Autodesk Inventor part; units mm, degrees
ref_plane "YZ Plane" through (0, 0, 0) normal (1, 0, 0) x (0, 1, 0)
ref_plane "XZ Plane" through (0, 0, 0) normal (0, 1, 0) x (-1, 0, 0)
ref_plane "XY Plane" through (0, 0, 0) normal (0, 0, 1) x (1, 0, 0)
sketch "Sketch1" plane through (0, 0, 0) normal (0, 1, 0) x (-1, 0, 0)
  line L0 (24.925, 14.925) -> (-24.925, 14.925)
  line L1 (-24.925, 14.925) -> (-24.925, -14.925)
  line L2 (-24.925, -14.925) -> (24.925, -14.925)
  line L3 (24.925, 14.925) -> (-24.925, -14.925) construction
  line L4 (-24.925, 14.925) -> (24.925, -14.925) construction
  line L5 (24.925, -14.925) -> (24.925, 14.925)
  line L6 (24.925, 5) -> (24.925, 14.925)
  point P0 (0, 0)
  dimension "d0" = 49.85
  dimension "d1" = 29.85
extrude "Extrusion1" add sketch "Sketch1" along normal blind 1.4
sketch "Sketch2" plane through (0, 0, 0) normal (0, -1, 0) x (1, 0, 0)
  point P0 (0, 0)
sketch "Sketch3" plane through (-24.925, 0, -14.925) normal (-1, 0, 0) x (0, 0, 1)
  point P0 (14.925, 0)
ref_plane "Work Plane1" through (0, 0, 0) normal (0, 1, 0) x (-1, 0, 0)
sketch "Sketch5" plane through (0, 0, 0) normal (0, 1, 0) x (-1, 0, 0)
  line L0 (-24.925, 14.925) -> (24.925, 14.925)
  line L1 (24.925, -14.925) -> (-24.925, -14.925)
  line L2 (24.925, 14.925) -> (24.925, -14.925)
  line L3 (-19.3821, 7.7039) -> (19.3821, 7.7039) construction
  line L4 (19.3821, 7.7039) -> (19.3821, -7.7039) construction
  line L5 (19.3821, -7.7039) -> (-19.3821, -7.7039) construction
  line L6 (-19.3821, -7.7039) -> (-19.3821, 7.7039) construction
  line L7 (-24.925, -14.925) -> (-24.925, 14.925)
  line L8 (-12.5833, 1.3105) -> (-16.2231, 1.3105)
  line L9 (-16.2231, 1.3105) -> (-16.2231, 3.7476)
  spline S0 degree 2 poles (-16.2231, 3.7476) (-16.2231, 4.8026) (-16.4552, 5.3301) (-16.8561, 5.3301) knots 0 0 0 1 2 2 2
  spline S1 degree 2 poles (-16.8561, 5.3301) (-17.3097, 5.3301) (-17.5524, 4.6866) (-17.5524, 3.6316) knots 0 0 0 1 2 2 2
  line L10 (-17.5524, 3.6316) -> (-17.5524, -2.8673)
  spline S2 degree 2 poles (-17.5524, -2.8673) (-17.5524, -3.8907) (-17.3097, -4.5131) (-16.8877, -4.5131) knots 0 0 0 1 2 2 2
  spline S3 degree 2 poles (-16.8877, -4.5131) (-16.4763, -4.5131) (-16.2231, -3.8907) (-16.2231, -2.7407) knots 0 0 0 1 2 2 2
  line L11 (-16.2231, -2.7407) -> (-16.2231, -0.9788)
  line L12 (-16.2231, -0.9788) -> (-12.5833, -0.9788)
  line L13 (-12.5833, -0.9788) -> (-12.5833, -1.5274)
  spline S4 degree 2 poles (-12.5833, -1.5274) (-12.5833, -3.7008) (-13.1952, -5.5154) (-15.3052, -6.8869) (-16.835, -6.8869) knots 0 0 0 1 2 3 3 3
  spline S5 degree 2 poles (-16.835, -6.8869) (-18.4386, -6.8869) (-20.517, -5.7264) (-21.1922, -3.6797) (-21.1922, -1.6224) knots 0 0 0 1 2 3 3 3
  line L14 (-21.1922, -1.6224) -> (-21.1922, 2.4711)
  spline S6 degree 2 poles (-21.1922, 2.4711) (-21.1922, 3.9797) (-20.9812, 5.4989) (-19.9578, 6.9021) (-18.1326, 7.7039) (-16.9405, 7.7039) knots 0 0 0 1 2 3 4 4 4
  spline S7 degree 2 poles (-16.9405, 7.7039) (-15.3369, 7.7039) (-13.2374, 6.459) (-12.5833, 4.6022) (-12.5833, 2.6399) knots 0 0 0 1 2 3 3 3
  line L15 (-12.5833, 2.6399) -> (-12.5833, 1.3105)
  line L16 (-11.2751, 7.4085) -> (-8.7008, 7.4085)
  spline S8 degree 2 poles (-8.7008, 7.4085) (-6.1266, 7.4085) (-4.3014, 7.0076) (-3.1515, 5.3723) (-3.1515, 3.5894) knots 0 0 0 1 2 3 3 3
  spline S9 degree 2 poles (-3.1515, 3.5894) (-3.1515, 1.9541) (-3.9638, 0.8252) (-5.156, 0.7092) knots 0 0 0 1 2 2 2
  spline S10 degree 2 poles (-5.156, 0.7092) (-4.0799, 0.4454) (-3.3308, -0.4513) (-3.1515, -1.2004) (-3.1515, -2.899) knots 0 0 0 1 2 3 3 3
  line L17 (-3.1515, -2.899) -> (-3.1515, -6.5915)
  line L18 (-3.1515, -6.5915) -> (-6.5381, -6.5915)
  line L19 (-6.5381, -6.5915) -> (-6.5381, -1.9389)
  spline S11 degree 2 poles (-6.5381, -1.9389) (-6.5381, -0.8206) (-6.8862, -0.2825) (-7.6353, -0.2825) knots 0 0 0 1 2 2 2
  line L20 (-7.6353, -0.2825) -> (-7.6353, -6.5915)
  line L21 (-7.6353, -6.5915) -> (-11.2751, -6.5915)
  line L22 (-11.2751, -6.5915) -> (-11.2751, 7.4085)
  line L23 (-7.6353, 5.0136) -> (-7.6353, 1.9013)
  spline S12 degree 2 poles (-7.6353, 1.9013) (-7.0234, 1.9013) (-6.5381, 2.239) (-6.5381, 3.1674) knots 0 0 0 1 2 2 2
  line L24 (-6.5381, 3.1674) -> (-6.5381, 3.9375)
  spline S13 degree 2 poles (-6.5381, 3.9375) (-6.5381, 4.6022) (-7.0128, 5.0136) (-7.6353, 5.0136) knots 0 0 0 1 2 2 2
  line L25 (4.5501, 7.4085) -> (6.639, -6.5915)
  line L26 (6.639, -6.5915) -> (2.9043, -6.5915)
  line L27 (2.9043, -6.5915) -> (2.7144, -4.07)
  line L28 (2.7144, -4.07) -> (1.4167, -4.07)
  line L29 (1.4167, -4.07) -> (1.2057, -6.5915)
  line L30 (1.2057, -6.5915) -> (-2.5712, -6.5915)
  line L31 (-2.5712, -6.5915) -> (-0.725, 7.4085)
  line L32 (-0.725, 7.4085) -> (4.5501, 7.4085)
  spline S14 degree 2 poles (2.6194, -1.5907) (2.3557, 0.783) (2.0708, 4.2857) knots 0 0 0 1 1 1
  spline S15 degree 2 poles (2.0708, 4.2857) (1.5222, 0.2661) (1.3745, -1.5907) knots 0 0 0 1 1 1
  line L33 (1.3745, -1.5907) -> (2.6194, -1.5907)
  line L34 (7.2615, 7.4085) -> (10.9329, 7.4085)
  spline S16 degree 2 poles (10.9329, 7.4085) (12.4205, 7.4085) (14.0241, 6.9443) (14.8259, 6.0581) (15.1108, 4.8026) (15.1108, 3.4944) knots 0 0 0 1 2 3 4 4 4
  line L35 (15.1108, 3.4944) -> (15.1108, 2.2706)
  spline S17 degree 2 poles (15.1108, 2.2706) (15.1108, 0.9307) (14.5516, -0.3036) (13.0746, -0.9577) (11.8824, -0.9577) knots 0 0 0 1 2 3 3 3
  line L36 (11.8824, -0.9577) -> (10.9013, -0.9577)
  line L37 (10.9013, -0.9577) -> (10.9013, -6.5915)
  line L38 (10.9013, -6.5915) -> (7.2615, -6.5915)
  line L39 (7.2615, -6.5915) -> (7.2615, 7.4085)
  line L40 (10.9013, 5.0136) -> (10.9013, 1.4477)
  spline S18 degree 2 poles (10.9013, 1.4477) (11.0595, 1.4371) (11.165, 1.4371) knots 0 0 0 1 1 1
  spline S19 degree 2 poles (11.165, 1.4371) (11.6714, 1.4371) (12.0618, 1.933) (12.0618, 2.7137) knots 0 0 0 1 2 2 2
  line L41 (12.0618, 2.7137) -> (12.0618, 3.8637)
  spline S20 degree 2 poles (12.0618, 3.8637) (12.0618, 4.5811) (11.6081, 5.0136) (10.9013, 5.0136) knots 0 0 0 1 2 2 2
  line L42 (19.6704, 7.4085) -> (19.4094, -2.7341)
  line L43 (19.4094, -2.7341) -> (17.8551, -2.7341)
  line L44 (17.8551, -2.7341) -> (17.5715, 7.4085)
  line L45 (17.5715, 7.4085) -> (19.6704, 7.4085)
  line L46 (19.5796, -6.5915) -> (17.6623, -6.5915)
  line L47 (17.6623, -6.5915) -> (17.6623, -4.6061)
  line L48 (17.6623, -4.6061) -> (19.5796, -4.6061)
  line L49 (19.5796, -4.6061) -> (19.5796, -6.5915)
  point P0 (0, 0)
  dimension "d13" = 29.85
  dimension "d14" = 49.85
  dimension "d16" = 38.7641
  dimension "d17" = 15.4078
  dimension "d18" = 7.2211
  dimension "d22" = 5.5429
extrude "Extrusion4" add sketch "Sketch5" against normal blind 0.4 contours L8 L9 S0 S1 L10 S2 S3 L11 L12 L13 S4 S5 L14 S6 S7 L15 | L16 S8 S9 S10 L17 L18 L19 S11 L20 L21 L22 | L25 L26 L27 L28 L29 L30 L31 L32 | L34 S16 L35 S17 L36 L37 L38 L39 | L42 L43 L44 L45 | L46 L47 L48 L49
sketch "Sketch6" plane through (0, 0, 0) normal (0, -1, 0) x (1, 0, 0)
  line L0 (-24.925, 14.925) -> (-24.925, -14.925)
  line L1 (24.925, 14.925) -> (-24.925, 14.925)
  line L2 (24.925, -14.925) -> (24.925, 14.925)
  line L3 (-24.925, -14.925) -> (24.925, -14.925)
  line L4 (-22.925, 10.925) -> (-22.925, -10.925)
  line L5 (-20.925, -12.925) -> (20.925, -12.925)
  line L6 (22.925, -10.925) -> (22.925, 10.925)
  line L7 (20.925, 12.925) -> (-20.925, 12.925)
  arc A0 (-20.925, 12.925) -> (-22.925, 10.925) centre (-20.925, 10.925) ccw
  arc A1 (-22.925, -10.925) -> (-20.925, -12.925) centre (-20.925, -10.925) ccw
  arc A2 (20.925, -12.925) -> (22.925, -10.925) centre (20.925, -10.925) ccw
  arc A3 (22.925, 10.925) -> (20.925, 12.925) centre (20.925, 10.925) ccw
  line L8 (-20.925, 12.525) -> (20.925, 12.525)
  arc A4 (22.525, 10.925) -> (20.925, 12.525) centre (20.925, 10.925) ccw
  line L9 (22.525, 10.925) -> (22.525, -10.925)
  arc A5 (20.925, -12.525) -> (22.525, -10.925) centre (20.925, -10.925) ccw
  line L10 (20.925, -12.525) -> (-20.925, -12.525)
  arc A6 (-22.525, -10.925) -> (-20.925, -12.525) centre (-20.925, -10.925) ccw
  line L11 (-22.525, -10.925) -> (-22.525, 10.925)
  arc A7 (-20.925, 12.525) -> (-22.525, 10.925) centre (-20.925, 10.925) ccw
  point P0 (0, 0)
  dimension "d23" = 2
  dimension "d24" = 2
  dimension "d25" = 0.4
extrude "Extrusion5" add sketch "Sketch6" along normal blind 0.4 contours A0 L7 A3 L6 A2 L5 A1 L4
equation "\"d18\" = 0.5 * d13 - 0.5 * d17"
equation "\"d22\" = 0.5 * d14 - 0.5 * d16"
properties part number "stamp5x3" material "PET Plastic"
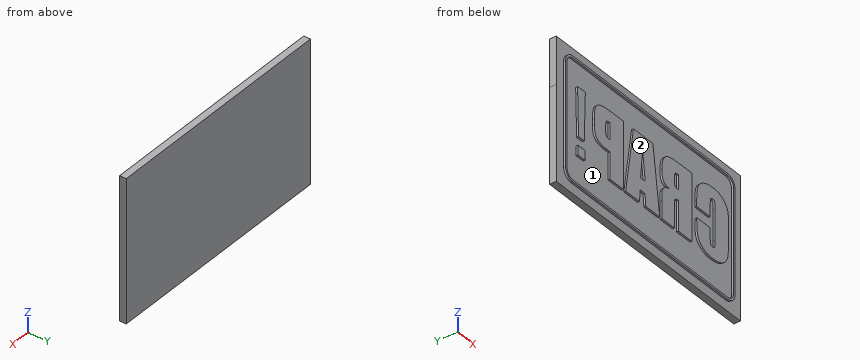
The model under review builds one solid part; all positions refer to its coordinate system, in mm. Face numbers are marked on the shaded views. Round coordinates to 2 decimals unless told otherwise and drop trailing zeros. Write each loop counter-clockwise with the first axis right and the second up, starting at its lowest first coordinate (ties: lowest second). Pieces come first, ordered by that corner, then holes. Notation, with made-up numbers: M 11,63 L 19,63 A16 ccw 19,84 Z; hole C -30.75,78.5 d2. An arc over 180 degrees is marked long. Answer as CSV lines item,"result". Start each with the question number.
Q1. Wall thickness on line 1 along Z through (x, y) = (-8.5, -0.05) (1 decimal); line 2 along Z through (x, y) = (-16.5, -0.1) (3 decimals); line 3 along Y through (x, z) = (-11, -7.5): over which ranges is each line inside the solid? List them lowest first.
Q2. Consider section B-B, the plane z = 11.75. Give the boundary of the cut face in (x, y) (3 decimals), then the cut area to 3 significant figures.
Q3. Clearance check with a flat-ended pin moving along its axis: P1, Ø0.9, axis at x = -11.5, z = 3, coming from the -Y side. State where the tip first meets the part, or that it passes through.
Q4. The part is to be moulded in two halves that separate along X. For the marked faces 1 and 2, say which applies: +X half, -X half, draft (parallel to the pull), parting line (faces both ways), or undercut.
Q5. Consider section A-A, the plane x = 12. Give the boundary of the cut face in (y, z) (3 decimals), then the cut area to 3 significant figures.
Result set:
1,line 1,"z = -12.9 to -12.5, -6.6 to 7.4, 12.5 to 12.9"
1,line 2,"z = -12.925 to -12.525, 12.525 to 12.925"
1,line 3,"y = 0 to 1.4"
2,outline,"M -24.925,0 L -22.747,0 L -22.747,-0.4 L -22.296,-0.4 L -22.296,0 L 22.296,0 L 22.296,-0.4 L 22.747,-0.4 L 22.747,0 L 24.925,0 L 24.925,1.4 L -24.925,1.4 Z"
2,area,"70.2 mm²"
3,P1,"stops at y = 0"
4,face 1,"undercut"
4,face 2,"draft"
5,outline,"M -0.4,-12.925 L 0,-12.925 L 0,-14.925 L 1.4,-14.925 L 1.4,14.925 L 0,14.925 L 0,12.925 L -0.4,12.925 L -0.4,12.525 L 0,12.525 L 0,-12.525 L -0.4,-12.525 Z"
5,area,"42.1 mm²"
